Work out the finished part from the listing and answer in its coordinate system (mm). Face numbers are marked on the shaded views. Round coordinates to 2 decimals unless told otherwise and drop trailing zeros. Loops run counter-clockwise (first coordinate to the right, second up) from the corner with the lowest first, then second, coordinate; pieces in that order, holes last. Notation, with made-up numbers: (11.5, -38.75) -> (48.5, -38.75) arc R32 cw to (48.5, -7.75) -> close; hole circle Ø7 at (82, -22). An arc over 180 degrees is marked (long way). Write item = value, one per line. Start each with the question number.
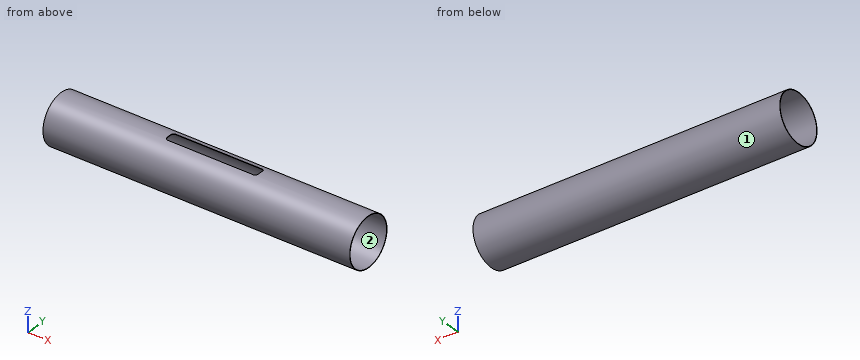
```python
from build123d import *

# Parameters (mm, degrees)
F0_R     = 22.225
F0_R_2   = 21.828125
F1_DEPTH = 139.7
F3_DEPTH = 25.4


with BuildPart() as f1:
    # F0 (on Right) → F1 (new body, symmetric)
    with BuildSketch(Plane.YZ):
        Circle(F0_R)
        Circle(F0_R_2, mode=Mode.SUBTRACT)
    extrude(amount=F1_DEPTH, both=True)

    # F2 (on Top) → F3 (cut)
    with BuildSketch(Plane.XY):
        with BuildLine():
            Line((38.989, 5.08), (-38.989, 5.08))
            ThreePointArc((-38.989, 5.08), (-40.785051, 4.336051), (-41.529, 2.54))
            Line((-41.529, 2.54), (-41.529, -2.54))
            ThreePointArc((-41.529, -2.54), (-40.785051, -4.336051), (-38.989, -5.08))
            Line((-38.989, -5.08), (38.989, -5.08))
            ThreePointArc((38.989, -5.08), (40.785051, -4.336051), (41.529, -2.54))
            Line((41.529, -2.54), (41.529, 2.54))
            ThreePointArc((41.529, 2.54), (40.785051, 4.336051), (38.989, 5.08))
        make_face()
    extrude(amount=F3_DEPTH, mode=Mode.SUBTRACT)


solid = f1.part
```
Item 1: Section D-D (x = 96) is taken. Determine the outline of the cut face in (y, z) (3 decimals).
Item 2: Flat-ended cylindrical pins translate along their axes: pin 1 (12 mm diameter, centred on x = 83.5, z = 11.5, fed in from +Y); pin 2 (12 mm diameter, centred on x = 15, y = 13.5, fed in from +Z); pin 3 (2 mm diameter, centred on x = -4, y = 6.5, fed in from -Z). Find the tip coordinate at first contact, or state that the pin passes through.
Item 3: Find the intervals of material crossed by line 1 along Z through (x, y) = (65, 0) (3 decimals); line 2 along Z through (x, y) = (35.5, -1.5); line 3 along Z through (x, y) = (-24, -8.5), in increasing order. Write a range as [from, to].
Item 4: The mould has two halves that part along Y. Classify the marked faces 1 and 2: pulls with the +Y half, pulls with the -Y half, needs draft (parallel to the pull), parting line crosses it, or undercut.
Item 5: Section A-A (z = 0) is taken. Determine the outline of the cut face in (x, y) (3 decimals), then the cut area to 3 significant figures.
Item 6: Section C-C (y = -14.5) is taken. Determine the outline of the cut face in (x, z), then the cut area to 3 significant figures.
Item 7: Section B-B (y = 0) is taken. Determine the outline of the cut face in (x, z) (3 decimals), then the cut area to 3 significant figures.
Worked answers:
q1.outline = circle Ø44.45 at (0, 0); hole circle Ø43.656 at (0, 0)
q2.pin_1 = 21.53
q2.pin_2 = 20.92
q2.pin_3 = -21.53
q3.line_1 = [-22.225, -21.828], [21.828, 22.225]
q3.line_2 = [-22.17, -21.78]
q3.line_3 = [-20.54, -20.11], [20.11, 20.54]
q4.face_1 = parting line crosses it
q4.face_2 = undercut
q5.outline = (-139.7, -22.225) -> (139.7, -22.225) -> (139.7, -21.828) -> (-139.7, -21.828) -> close; (-139.7, 21.828) -> (139.7, 21.828) -> (139.7, 22.225) -> (-139.7, 22.225) -> close
q5.area = 222 mm2
q6.outline = (-139.7, -16.84) -> (139.7, -16.84) -> (139.7, -16.32) -> (-139.7, -16.32) -> close; (-139.7, 16.32) -> (139.7, 16.32) -> (139.7, 16.84) -> (-139.7, 16.84) -> close
q6.area = 295 mm2
q7.outline = (-139.7, -22.225) -> (139.7, -22.225) -> (139.7, -21.828) -> (-139.7, -21.828) -> close; (-139.7, 21.828) -> (-41.529, 21.828) -> (-41.529, 22.225) -> (-139.7, 22.225) -> close; (41.529, 21.828) -> (139.7, 21.828) -> (139.7, 22.225) -> (41.529, 22.225) -> close
q7.area = 189 mm2
